Source: CAD feature listing. Evaluate the final solid. Frame: model axes, mm. A direction names the side the tool comes from. Give positions to 0.01 mm unless a question says otherwise; leave off trailing zeros. Write each loop counter-clockwise with the first axis right and the second up, starting at its lowest first coordinate (ties: lowest second). Pieces come first, ordered by that corner, then holes. Notation, with made-up numbers: (75.5, 1) -> (126.5, 1) arc R17 ccw to (126.5, 26) -> close; hole circle Ø9 at (-27, -27). An arc over 180 degrees is marked (long way). Answer as a JSON object with one key per item and string values. Group by question number.
Item 1: Section query C-C on x = 14. Return the cut outline in (y, z).
Item 2: Pull-direction query (X, two-part tool) for faces 1 (the face through (104.5, 5, 1)), 2 (the face through (-1.9, 3.6, 2)), 3 (the face through (33.5, 4, 4)); classes: pulls with the +X half, pulls with the -X half, needs draft (parallel to the pull), parting line crosses it, or undercut.
Item 3: Section query B-B on z = 4.2. Return the cut outline in (x, y).
Item 4: First-contact query: pin 1 Ø0.9 at (y, z) = (5, 4) entering from +X; pin 2 Ø0.9 at (y, z) = (4.5, 3) entering from -X; pin 3 Ø3.5 at (x, y) = (-5, 5) entering from +Z. Flat tips, straight axial feed; report the tip coordinate or a pass-through.
Item 5: Access query for faces 4 (the face through (17, 5, 2)), 5 (the face through (48, 0, 1)), 6 (the face through (0, 5, 3)). Directions: +Z, -Z, +X, -X, +Y, -Y. A direction counts if a zero-diameter tool reaches every point of the face in a straight line with its end or side. Return the directions, or none.
Item 6: Ray query, probe 1 along X at (y, z) = (4.5, 1.2); probe 2 along Y at (x, z) = (-3.5, 1.45); probe 3 along X at (y, z) = (4, 2.25). Return the intervals inside material, ascending. Write a range as from..to.
Item 7: Section query A-A on y = 4.5. Return the cut outline in (x, z).
Autodesk Inventor part; units mm, degrees
ref_plane "YZ Plane" through (0, 0, 0) normal (1, 0, 0) x (0, 1, 0)
ref_plane "XZ Plane" through (0, 0, 0) normal (0, 1, 0) x (-1, 0, 0)
ref_plane "XY Plane" through (0, 0, 0) normal (0, 0, 1) x (1, 0, 0)
sketch "Sketch1" plane through (0, 0, 0) normal (0, 0, 1) x (1, 0, 0)
  line L0 (0, 0) -> (97.5, 0)
  line L1 (97.5, 0) -> (97.5, 9)
  line L2 (97.5, 9) -> (0, 9)
  line L3 (0, 9) -> (0, 0)
  dimension "d2" = 97.5
  dimension "d3" = 9
extrude "Extrusion1" add sketch "Sketch1" along normal blind 5
sketch "Sketch2" plane through (0, 0, 5) normal (0, 0, 1) x (1, 0, 0)
  line L0 (0, 0) -> (97.5, 0)
  line L1 (97.5, 0) -> (97.5, 9)
  line L2 (0, 9) -> (0, 0)
  line L3 (2, 0) -> (32.5, 0)
  line L4 (32.5, 0) -> (32.5, 9)
  line L5 (32.5, 9) -> (2, 9)
  line L6 (2, 9) -> (2, 0)
  line L7 (33.5, 9) -> (64, 9)
  line L8 (64, 9) -> (64, 0)
  line L9 (64, 0) -> (33.5, 0)
  line L10 (33.5, 0) -> (33.5, 9)
  line L11 (65, 0) -> (95.5, 0)
  line L12 (95.5, 0) -> (95.5, 9)
  line L13 (95.5, 9) -> (65, 9)
  line L14 (65, 9) -> (65, 0)
  line L15 (97.5, 9) -> (0, 9)
  dimension "d5" = 30.5
  dimension "d6" = 2
  dimension "d7" = 2
  dimension "d8" = 30.5
  dimension "d9" = 30.5
  dimension "d10" = 1
extrude "Extrusion2" cut sketch "Sketch2" against normal blind 3 contours L6 L5 L4 L0 | L10 L7 L8 L0 | L14 L13 L12 L0
sketch "Sketch3" plane through (0, 0, 0) normal (-1, 0, 0) x (0, 0, 1)
  line L0 (0, 9) -> (0, 0)
  line L1 (0, 0) -> (5, 0)
  line L2 (0, 9) -> (2, 9)
  line L3 (2, 9) -> (2, 0)
  line L4 (2, 0) -> (0, 0)
  line L5 (0, 0) -> (0, 9)
  dimension "d13" = 2
extrude "Extrusion3" add sketch "Sketch3" along normal blind 7
sketch "Sketch5" plane through (97.5, 0, 0) normal (1, 0, 0) x (0, 0, -1)
  line L0 (0, 0) -> (-5, 0)
  line L1 (0, 9) -> (-2, 9)
  line L2 (-2, 9) -> (-2, 0)
  line L3 (-2, 0) -> (0, 0)
  line L4 (0, 0) -> (0, 9)
  dimension "d22" = 2
extrude "Extrusion5" add sketch "Sketch5" along normal blind 7
sketch "Sketch7" plane through (0, 0, 2) normal (0, 0, 1) x (1, 0, 0)
  line L0 (-7, 0) -> (-7, 9)
  line L1 (0, 0) -> (-7, 0)
  line L2 (97.5, 0) -> (97.5, 9)
  line L3 (97.5, 0) -> (104.5, 0)
  line L4 (104.5, 9) -> (104.5, 0)
  line L5 (97.5, 9) -> (104.5, 9)
  point P0 (-3.5, 4.5)
  point P1 (101, 4.5)
  dimension "d31" = 3.5
  dimension "d32" = 4.5
  dimension "d33" = 4.5
  dimension "d34" = 3.5
hole "Hole1" at (-3.5, 4.5, 2) at (101, 4.5, 2) direction (0, 0, -1) diameter 3 end through all
ref_plane "Work Plane1" through (33.5, 4.5, 2) normal (0, -1, 0) x (1, 0, 0)
fillet "Fillet1" radius 3 4 edges at (104.5, 0, 1) (104.5, 9, 1) (-7, 0, 1) (-7, 9, 1)
properties part number "base_corner" material "ABS Plastic"
Worked answers:
{
 "1": {"outline": "(0, 0) -> (9, 0) -> (9, 2) -> (0, 2) -> close"},
 "2": {"face 1": "pulls with the +X half", "face 2": "needs draft", "face 3": "undercut"},
 "3": {"outline": "(0, 0) -> (2, 0) -> (2, 9) -> (0, 9) -> close; (32.5, 0) -> (33.5, 0) -> (33.5, 9) -> (32.5, 9) -> close; (64, 0) -> (65, 0) -> (65, 9) -> (64, 9) -> close; (95.5, 0) -> (97.5, 0) -> (97.5, 9) -> (95.5, 9) -> close"},
 "4": {"pin 1": "x = 97.5", "pin 2": "x = 0", "pin 3": "z = 2"},
 "5": {"face 4": "+Z, +Y, -Y", "face 5": "+Z, -Z, +X, -X, -Y", "face 6": "+Z, -X, +Y, -Y"},
 "6": {"probe 1": "-7..-5, -2..99.5, 102.5..104.5", "probe 2": "0..3, 6..9", "probe 3": "0..2, 32.5..33.5, 64..65, 95.5..97.5"},
 "7": {"outline": "(-7, 0) -> (-5, 0) -> (-5, 2) -> (-7, 2) -> close; (-2, 0) -> (99.5, 0) -> (99.5, 2) -> (97.5, 2) -> (97.5, 5) -> (95.5, 5) -> (95.5, 2) -> (65, 2) -> (65, 5) -> (64, 5) -> (64, 2) -> (33.5, 2) -> (33.5, 5) -> (32.5, 5) -> (32.5, 2) -> (2, 2) -> (2, 5) -> (0, 5) -> (0, 2) -> (-2, 2) -> close; (102.5, 0) -> (104.5, 0) -> (104.5, 2) -> (102.5, 2) -> close"}
}
